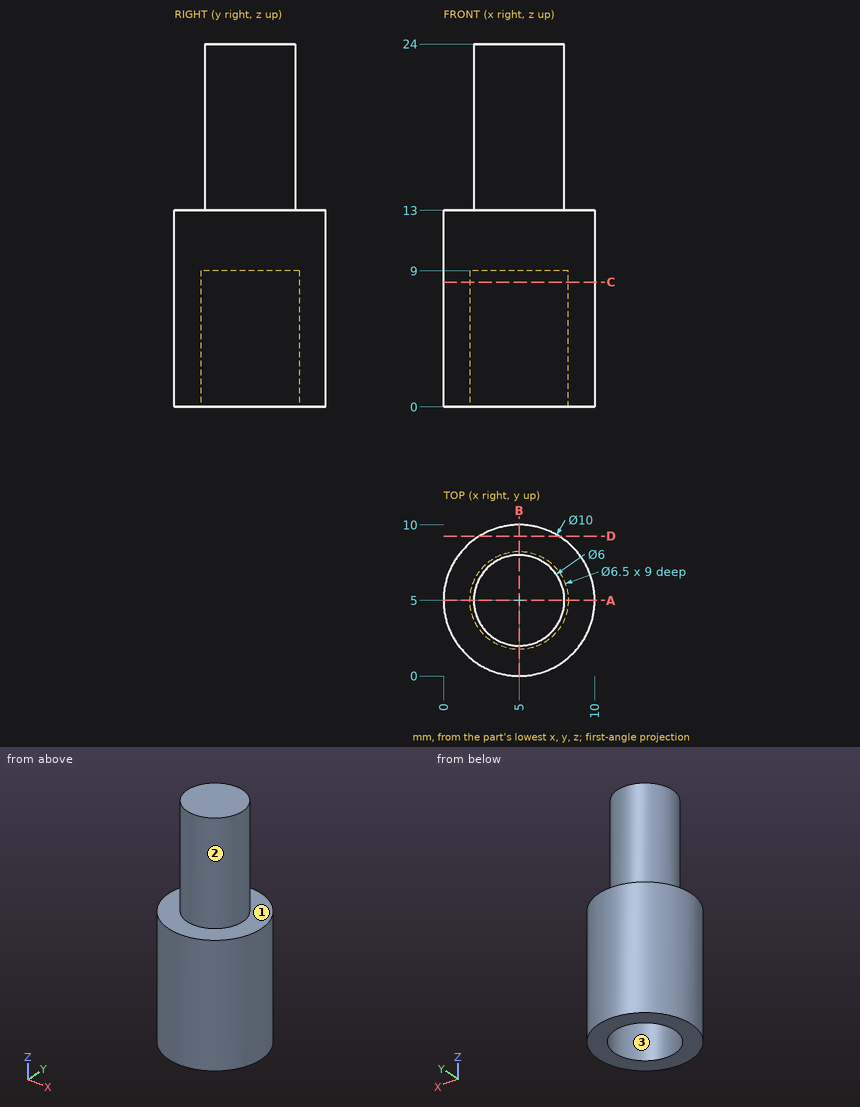
Input: dimensioned drawing with shaded views. Units: mm. Origin: part minimum x, y, z. Round coordinates to 2 decimals unless told otherwise and drop trailing zeros. Order: outer loops, then holes, each group sorted by start corner. A loop starts at its lowest first (then second) coordinate and runs counter-clockwise, first axis right, second up.
1. Mould query, pull axis Y, two halves, no side actions, for the marked faces 1, 2 and 3. Classes: released by +Y, released by -Y, zero draft, split by the parting line, or undercut.
The answers:
face 1: zero draft
face 2: split by the parting line
face 3: undercut
2. Cut plane D-D, the plane y = 9.25. Output: boundary loops of the cut face in (x, z), then the cut area to 3 significant figures.
The answers:
outline: (2.37, 0) - (7.63, 0) - (7.63, 13) - (2.37, 13) - close
area: 68.5 mm2
3. Cut plane A-A, the plane y = 5. Output: boundary loops of the cut face in (x, z).
The answers:
outline: (0, 0) - (1.75, 0) - (1.75, 9) - (8.25, 9) - (8.25, 0) - (10, 0) - (10, 13) - (8, 13) - (8, 24) - (2, 24) - (2, 13) - (0, 13) - close
4. Cut plane C-C, the plane z = 8.25. Output: boundary loops of the cut face in (x, y).
The answers:
outline: circle Ø10 at (5, 5); hole circle Ø6.5 at (5, 5)
5. Pin query (flat end, axial travel): P1, Ø5, axis at y = 2.5, z = 17.5, coming from the -X side; P2, Ø4, axis at x = 7.5, z = 12, coming from the +Y side; P3, Ø2, axis at y = 2, z = 3, coming from the +X side. Return the tip coordinate at first contact, or that it passes through.
The answers:
P1: stops at x = 2
P2: stops at y = 9.97
P3: stops at x = 9.58
6. Material intervals for line 1 (Y direction, x = 5, z = 5); line 2 (Z direction, x = 9.75, y = 4.5); line 3 (Z direction, x = 7.75, y = 4.25), sorted ascending.
The answers:
line 1: y = 0 to 1.75, 8.25 to 10
line 2: z = 0 to 13
line 3: z = 9 to 24
